Work out the finished part from the listing and answer in its coordinate system (mm). Give positions to 0.01 mm unless a question says otherwise; leave off trailing zeros. Order: outer loops, then holes, each group sorted by start corner. A loop starts at its lowest first (then second) coordinate and runs counter-clockwise, first axis right, second up. Notation, with made-up numbers: (-18, 57.25) - (21, 57.25) arc R17 ccw to (21, 66.25) - close; hole circle Ø10 at (-12, 27.25). An arc over 180 degrees is marked (long way). Write each question's results on one line, items separated by ' | '.
from build123d import *

# Parameters (mm, degrees)
ESQUISSE1_W             = 180
ESQUISSE1_H             = 790
BOSS_EXTRU_1_DEPTH      = 5
ESQUISSE2_W             = 130
ESQUISSE2_H             = 180
ENL_V_MAT_EXTRU_1_DEPTH = 406.154291598
ESQUISSE3_W             = 180
ESQUISSE3_H             = 100
ENL_V_MAT_EXTRU_2_DEPTH = 5
ESQUISSE4_R             = 22.583693943
ESQUISSE4_W             = 39.272250948
ESQUISSE4_H             = 13.375687181
ENL_V_MAT_EXTRU_3_DEPTH = 10
ESQUISSE6_R             = 1.5
ESQUISSE6_W             = 43.78333401
ESQUISSE6_H             = 30.495607997
ESQUISSE6_W_2           = 33.572233796
ESQUISSE6_H_2           = 23.130308998
ENL_V_MAT_EXTRU_4_DEPTH = 10
ESQUISSE7_R             = 1.5
ESQUISSE7_W             = 44.788511225
ESQUISSE7_H             = 29.879964446
ESQUISSE7_W_2           = 33.612496144
ESQUISSE7_H_2           = 23.111104951
ENL_V_MAT_EXTRU_5_DEPTH = 10


with BuildPart() as part:
    # Esquisse1 → Boss.-Extru.1 (new body)
    with BuildSketch(Plane.XY):
        Rectangle(ESQUISSE1_W, ESQUISSE1_H)
    extrude(amount=BOSS_EXTRU_1_DEPTH)

    # Esquisse2 → Enlèv. mat.-Extru.1 (cut, through all)
    with BuildSketch(Plane.XY.offset(5)):
        Rectangle(ESQUISSE2_W, ESQUISSE2_H)
    extrude(amount=-ENL_V_MAT_EXTRU_1_DEPTH, mode=Mode.SUBTRACT)

    # Esquisse3 → Enlèv. mat.-Extru.2 (cut)
    with BuildSketch(Plane.XY.offset(5)):
        with Locations((0, -345)):
            Rectangle(ESQUISSE3_W, ESQUISSE3_H)
    extrude(amount=-ENL_V_MAT_EXTRU_2_DEPTH, mode=Mode.SUBTRACT)

    # Esquisse4 → Enlèv. mat.-Extru.3 (cut)
    with BuildSketch(Plane.XY.offset(5)):
        with Locations((-5, 315.089745962)):
            Circle(ESQUISSE4_R)
        with Locations((-5, 251.402324932)):
            Rectangle(ESQUISSE4_W, ESQUISSE4_H)
    extrude(amount=-ENL_V_MAT_EXTRU_3_DEPTH, mode=Mode.SUBTRACT)

    # Esquisse6 → Enlèv. mat.-Extru.4 (cut)
    with BuildSketch(Plane.XY.offset(5)):
        with Locations((-12.09, -189.669997694)):
            Circle(ESQUISSE6_R)
        with Locations((18.36, -189.669997694)):
            Circle(ESQUISSE6_R)
        with Locations((18.36, -161.269997694)):
            Circle(ESQUISSE6_R)
        with Locations((-12.09, -161.269997694)):
            Circle(ESQUISSE6_R)
        with Locations((1.217144904, -210.087843678)):
            Rectangle(ESQUISSE6_W, ESQUISSE6_H)
        with Locations((3.160802391, -175.467764734)):
            Rectangle(ESQUISSE6_W_2, ESQUISSE6_H_2)
    extrude(amount=-ENL_V_MAT_EXTRU_4_DEPTH, mode=Mode.SUBTRACT)

    # Esquisse7 → Enlèv. mat.-Extru.5 (cut)
    with BuildSketch(Plane.XY.offset(5)):
        with Locations((62.66, 315.355)):
            Circle(ESQUISSE7_R)
        with Locations((32.21, 315.355)):
            Circle(ESQUISSE7_R)
        with Locations((32.21, 286.955)):
            Circle(ESQUISSE7_R)
        with Locations((62.66, 286.955)):
            Circle(ESQUISSE7_R)
        with Locations((46.118085251, 266.662403555)):
            Rectangle(ESQUISSE7_W, ESQUISSE7_H)
        with Locations((47.453751928, 301.139447525)):
            Rectangle(ESQUISSE7_W_2, ESQUISSE7_H_2)
    extrude(amount=-ENL_V_MAT_EXTRU_5_DEPTH, mode=Mode.SUBTRACT)


solid = part.part
1. A cutting plane is placed at A-A, the plane x = -42.5. Write down the section's boundary in (y, z).
Answer list:
outline: (-295, 0) - (-90, 0) - (-90, 5) - (-295, 5) - close; (90, 0) - (395, 0) - (395, 5) - (90, 5) - close
2. A cutting plane is placed at C-C, the plane z = 3. State how many separate pieces and enclosed holes the cut face has, then the cut area to 3 significant figures.
Answer list:
separate pieces: 1 | enclosed holes: 15 | area: 94,400 mm^2
3. Determine the mould class of faces 1 (the face through (-9.896, 293.043, 2.535)), 2 (the face through (-1, 131, 5)) for opening direction X: +X half, -X half, draft (parallel to the pull), parting line (faces both ways), or undercut.
Answer list:
face 1: undercut | face 2: draft
4. A cutting plane is placed at B-B, the plane y = 41.5. Write down the section's boundary in (x, z), then the cut area to 3 significant figures.
Answer list:
outline: (-90, 0) - (-65, 0) - (-65, 5) - (-90, 5) - close; (65, 0) - (90, 0) - (90, 5) - (65, 5) - close | area: 250 mm^2
5. Straight lines are drawn through the part: line 1 (Y direction, x = 32.21, z = 1.55) (3 decimals); line 2 (Y direction, x = 63, z = 2.3) (3 decimals); line 3 (X direction, y = -214, z = 3.15). For each, find the intervals that lie inside material, in ascending order. Write a range as [from, to].
Answer list:
line 1: [-295, -90], [90, 251.722], [281.602, 285.455], [288.455, 289.584], [312.695, 313.855], [316.855, 395] | line 2: [-295, -90], [90, 251.722], [281.602, 285.494], [288.416, 289.584], [312.695, 313.894], [316.816, 395] | line 3: [-90, -20.67], [23.11, 90]
